```python
from build123d import *

# Parameters (mm, degrees)
BOSS_EXTRUDE1_DEPTH   = 12.7
SKETCH2_R             = 7.62
CUT_EXTRUDE1_DEPTH    = 16.875
FILLET1_R             = 3.175
F_4_CLEARANCE_HOLE1_D = 2.9464
M2_CLEARANCE_HOLE1_D  = 2.2
CUT_EXTRUDE2_DEPTH    = 16.875
FILLET2_R             = 0.508


with BuildPart() as part:
    # Sketch1 → Boss-Extrude1 (new body, symmetric)
    with BuildSketch(Plane(origin=(0, 0, 0), x_dir=(0, 0, -1), z_dir=(1, 0, 0))):
        Polygon((0, 38.1), (0, 0), (15.875, 0), (15.875, 3.175), (3.175, 3.175), (3.175, 38.1), align=None)
    extrude(amount=BOSS_EXTRUDE1_DEPTH, both=True)

    # Sketch2 → Cut-Extrude1 (cut, through all)
    with BuildSketch(Plane.XY):
        with Locations((0, 25.908)):
            Circle(SKETCH2_R)
    extrude(amount=-CUT_EXTRUDE1_DEPTH, mode=Mode.SUBTRACT)

    # Fillet1
    fillet1_edges = [part.edges().sort_by_distance(p)[0] for p in [
        (12.7, 1.5875, -15.875),
        (12.7, 38.1, -1.5875),
        (-12.7, 1.5875, -15.875),
        (-12.7, 38.1, -1.5875),
    ]]
    fillet(fillet1_edges, radius=FILLET1_R)

    # #4 Clearance Hole1 (through all)
    with Locations(Plane(origin=(0, 3.175, 0), x_dir=(1, 0, 0), z_dir=(0, 1, 0))):
        with Locations((-9.525, 6.35), (0, 12.7), (9.525, 6.35)):
            Hole(F_4_CLEARANCE_HOLE1_D / 2)

    # M2 Clearance Hole1 (through all)
    with Locations(Plane(origin=(32.851265871, 6.645872946, 0), x_dir=(0, 1, 0), z_dir=(0, 0, 1))):
        with Locations((19.262127054, 22.351265871), (19.262127054, 43.351265871)):
            Hole(M2_CLEARANCE_HOLE1_D / 2)

    # Sketch7 → Cut-Extrude2 (cut, through all)
    with BuildSketch(Plane.XY):
        with BuildLine():
            Line((-9.525, 20.828), (-9.525, 4.7625))
            Line((-9.525, 4.7625), (9.525, 4.7625))
            Line((9.525, 4.7625), (9.525, 20.828))
            ThreePointArc((9.525, 20.828), (0, 15.113), (-9.525, 20.828))
        make_face()
    extrude(amount=-CUT_EXTRUDE2_DEPTH, mode=Mode.SUBTRACT)

    # Fillet2
    fillet2_edges = [part.edges().sort_by_distance(p)[0] for p in [
        (-9.525, 20.828, -1.5875),
        (9.525, 20.828, -1.5875),
        (9.525, 4.7625, -1.5875),
        (-9.525, 4.7625, -1.5875),
    ]]
    fillet(fillet2_edges, radius=FILLET2_R)


solid = part.part
```
The model under review builds one solid part; all positions refer to its coordinate system, in mm. A direction names the side the tool comes from. Coordinates: 2 decimals unless noted, no trailing zeros. Write each loop counter-clockwise with the first axis right and the second up, starting at its lowest first coordinate (ties: lowest second). Pieces come first, ordered by that corner, then holes.
1) We need section A-A on x = 0. State the section outline as (y, z) points (1 decimal).
2) The part is to be moulded in two halves that separate along X. For faces 3 (the face through (11.75, 37.19, -1.57)), 4 (the face through (0.14, 15.114, -1.565)), 5 (the face through (0, 0, -8)), 6 (the face through (0, 4.762, -2)), say which applies: pulls with the +X half, pulls with the -X half, needs draft (parallel to the pull), parting line crosses it, or undercut.
3) Machinability: for faces 1 (the face through (-8.4, 1.6, -7.3)), 2 (the face through (-9.19, 19.57, -1.61)), which of the approach directions +Z, -Z, +X, -X, +Y, -Y give a long, thin tool a straight path to every point of the face, cutting with its end or side? Answer none if there is none.
4) To check wall thickness, follow probe 1 along X at (y, z) = (1.9, -6.35); probe 2 along Y at (x, z) = (-4, -1.75); probe 3 along Y at (x, z) = (10.25, -8) (3 decimals). State the ranges of each line that lie inside material, in increasing order.
5) We need section D-D on x = -10.5. State the section outline as (y, z) points (3 decimals), then the cut area to 3 significant figures.
6) We need section C-C on x = 5.75. State the section outline as (y, z) points (1 decimal), then the cut area to 3 significant figures.
7) Clearance check with flat-ended pins moving along their axes: pin 1 Ø2 at (x, y) = (-9, 17) entering from -Z (3 decimals); pin 2 Ø1.5 at (x, z) = (2.5, -5.5) entering from +Y (3 decimals). State where each tip first meets the part, or that it passes through.
8) We need section B-B on y = 7. State the section outline as (x, z) points (3 decimals), then the cut area to 3 significant figures.
Answer list:
1. outline: (0, -15.9) - (3.2, -15.9) - (3.2, -14.2) - (0, -14.2) - close; (0, -11.2) - (3.2, -11.2) - (3.2, -3.2) - (4.8, -3.2) - (4.8, 0) - (0, 0) - close; (15.1, -3.2) - (18.3, -3.2) - (18.3, 0) - (15.1, 0) - close; (33.5, -3.2) - (38.1, -3.2) - (38.1, 0) - (33.5, 0) - close
2. face 3: pulls with the +X half
2. face 4: undercut
2. face 5: needs draft
2. face 6: undercut
3. face 1: +Y, -Y
3. face 2: +Z, -Z
4. probe 1: x = -12.7 to -11, -8.05 to 8.05, 11 to 12.7
4. probe 2: y = 0 to 4.76, 15.88 to 19.42, 32.39 to 38.1
4. probe 3: y = 0 to 3.175
5. outline: (0, -15.722) - (3.175, -15.722) - (3.175, -7.454) - (0, -7.454) - close; (0, -5.246) - (3.175, -5.246) - (3.175, -3.175) - (24.808, -3.175) - (24.808, 0) - (0, 0) - close; (27.008, -3.175) - (37.947, -3.175) - (37.947, 0) - (27.008, 0) - close
5. area: 146 mm2
6. outline: (0, -15.9) - (3.2, -15.9) - (3.2, -3.2) - (4.8, -3.2) - (4.8, 0) - (0, 0) - close; (16.8, -3.2) - (20.9, -3.2) - (20.9, 0) - (16.8, 0) - close; (30.9, -3.2) - (38.1, -3.2) - (38.1, 0) - (30.9, 0) - close
6. area: 91.4 mm2
7. pin 1: stops at z = -3.175
7. pin 2: stops at y = 3.175
8. outline: (-12.7, -3.175) - (-9.525, -3.175) - (-9.525, 0) - (-12.7, 0) - close; (9.525, -3.175) - (12.7, -3.175) - (12.7, 0) - (9.525, 0) - close
8. area: 20.2 mm2
